from build123d import *

# Parameters (mm, degrees)
F0_W     = 13.5
F0_H     = 7
F1_DEPTH = 40


with BuildPart() as f1:
    # F0 (on Front) → F1 (new body)
    with BuildSketch(Plane.XZ):
        Polygon((-10, 0), (0, 0), (10, 0), (23.470384, 13.470384), (44.683588, -7.742819), (51.754655, -0.671751), (20, 31.082904), (0, 31.082904), (-20, 31.082904), (-51.754655, -0.671751), (-44.683588, -7.742819), (-23.470384, 13.470384), align=None)
        with Locations((0, 17.262155)):
            Rectangle(F0_W, F0_H, mode=Mode.SUBTRACT)
    extrude(amount=F1_DEPTH)


solid = f1.part
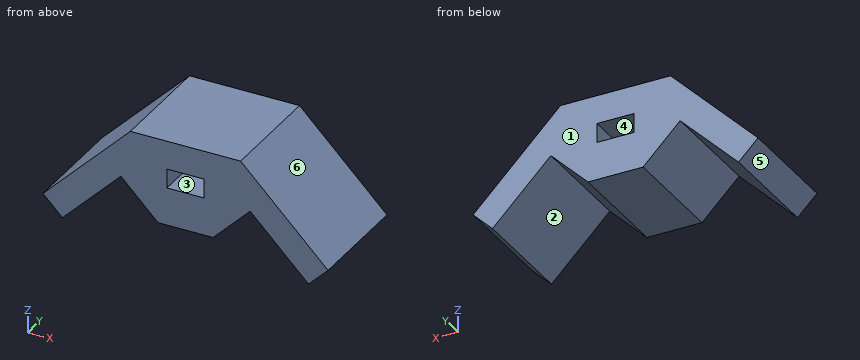
Geometry: final body of the model. Coordinates: model frame, mm. Face numbers are marked on the shaded views. A direction names the side the tool comes from. Give positions to 0.01 mm unless a question says otherwise; leave off trailing zeros. Loops run counter-clockwise (first coordinate to the right, second up) from the corner with the lowest first, then second, coordinate; pieces in that order, holes last. Notation, with made-up numbers: M 83.5,33.25 L 89.5,33.25 A7 ccw 89.5,43.25 Z; hole C 65.25,45.5 d2. An arc over 180 degrees is marked long. Put each result on its own line as item: value.
1) Cut plane C-C, the plane z = 11. Return the cut outline in (x, y), plus the area to 3 significant figures.
Computed values:
outline: M -40.08,-40 L -25.94,-40 L -25.94,0 L -40.08,0 Z; M -21,-40 L 21,-40 L 21,0 L -21,0 Z; M 25.94,-40 L 40.08,-40 L 40.08,0 L 25.94,0 Z
area: 2,810 mm^2
2) Cut plane B-B, the plane y = -13. Return the cut outline in (x, z), plus the area to 3 significant figures.
Computed values:
outline: M -51.75,-0.67 L -44.68,-7.74 L -23.47,13.47 L -10,0 L 10,0 L 23.47,13.47 L 44.68,-7.74 L 51.75,-0.67 L 20,31.08 L -20,31.08 Z; hole M -6.75,13.76 L 6.75,13.76 L 6.75,20.76 L -6.75,20.76 Z
area: 1,870 mm^2
3) Cut plane D-D, the plane z = 18. Return the cut outline in (x, y), plus the area to 3 significant figures.
Computed values:
outline: M -33.08,-40 L -6.75,-40 L -6.75,0 L -33.08,0 Z; M 6.75,-40 L 33.08,-40 L 33.08,0 L 6.75,0 Z
area: 2,110 mm^2
4) Cut plane A-A, the plane x = 1. Return the cut outline in (y, z).
Computed values:
outline: M -40,0 L 0,0 L 0,13.76 L -40,13.76 Z; M -40,20.76 L 0,20.76 L 0,31.08 L -40,31.08 Z
5) Reachability of the marked faces 1 and 2 from +Z, -Z, +X, -X, +Y, -Y: full face, straight path, thin tool, end or side. Return the list, or none.
Computed values:
face 1: +Z, -Z, +X, -X, +Y
face 2: -Z, +Y, -Y
6) Material intervals for L1, parallel to X at y = -36, z = 12; L2, parallel to X at y = -23, z = 11; L3, parallel to Z at x = -3, y = -20, sorted ascending. Write a range as from..to.
Computed values:
L1: x = -39.08..-24.94, -22..22, 24.94..39.08
L2: x = -40.08..-25.94, -21..21, 25.94..40.08
L3: z = 0..13.76, 20.76..31.08
7) Mould query, pull axis Z, two halves, no side actions, for the marked faces 3, 4, 5 and 6. Classes: released by +Z, released by -Z, zero draft, split by the parting line, or undercut.
Computed values:
face 3: undercut
face 4: undercut
face 5: released by -Z
face 6: released by +Z
8) First-contact query: P1, Ø6, axis at y = -10, z = 2.5, coming from the -X side; P2, Ø4, axis at y = -9, z = 4.5, coming from the -X side; P3, Ø4, axis at y = -21.5, z = -2.5, coming from the -X side; P4, Ø10, axis at x = -7.5, z = 24.5, coming from the +Y side. Flat tips, straight axial feed; report the tip coordinate or a pass-through.
Computed values:
P1: stops at x = -51.58
P2: stops at x = -48.58
P3: stops at x = -51.75
P4: stops at y = 0
